Here's how the part is built. I have some questions about the finished solid (model axes, mm). Face numbers are marked on the shaded views. Coordinates: 2 decimals unless noted, no trailing zeros. Loops run counter-clockwise (first coordinate to the right, second up) from the corner with the lowest first, then second, coordinate; pieces in that order, holes last.
from build123d import *

# Parameters (mm, degrees)
F1_DEPTH  = 10.16
F2_W      = 208.28
F2_H      = 116.84
F3_DEPTH  = 0.254
F4_R      = 9.807477688
F4_R_2    = 8.537478745
F5_DEPTH  = 0.508
F6_DEPTH  = 0.254
F7_W      = 15.5448025422
F7_H      = 2.0574
F8_DEPTH  = 1.27
F9_DEPTH  = 0.254
F10_R     = 2.0193
F11_DEPTH = 0.762
F13_DEPTH = 2.54
F14_R     = 1.5445798635
F15_DEPTH = 2.54
F17_DEPTH = 76.2
F19_DEPTH = 0.762
F20_R     = 5.191457902
F20_R_2   = 3.4134577513
F21_DEPTH = 0.762
F22_DEPTH = 0.762
F23_R     = 2.6550671555
F24_DEPTH = 0.508


with BuildPart() as f1:
    # F0 (on Top) → F1 (new body)
    with BuildSketch(Plane.XY):
        with BuildLine():
            Line((-133.35, 0), (-133.35, -50.8))
            Line((-133.35, -50.8), (-133.35, -57.15))
            ThreePointArc((-133.35, -57.15), (-131.4901280605, -61.6401280605), (-127, -63.5))
            Line((-127, -63.5), (-120.65, -63.5))
            Line((-120.65, -63.5), (0, -63.5))
            Line((0, -63.5), (0, 0))
            Line((0, 0), (-133.35, 0))
        make_face()
        with BuildLine():
            Line((-133.35, 50.8), (-133.35, 0))
            Line((-133.35, 0), (0, 0))
            Line((0, 0), (0, 63.5))
            Line((0, 63.5), (-120.65, 63.5))
            Line((-120.65, 63.5), (-127, 63.5))
            ThreePointArc((-127, 63.5), (-131.4901280605, 61.6401280605), (-133.35, 57.15))
            Line((-133.35, 57.15), (-133.35, 50.8))
        make_face()
        with BuildLine():
            Line((0, 63.5), (0, 0))
            Line((0, 0), (0, -63.5))
            Line((0, -63.5), (120.65, -63.5))
            Line((120.65, -63.5), (127, -63.5))
            ThreePointArc((127, -63.5), (131.4901280605, -61.6401280605), (133.35, -57.15))
            Line((133.35, -57.15), (133.35, -50.8))
            Line((133.35, -50.8), (133.35, 50.8))
            Line((133.35, 50.8), (133.35, 57.15))
            ThreePointArc((133.35, 57.15), (131.4901280605, 61.6401280605), (127, 63.5))
            Line((127, 63.5), (120.65, 63.5))
            Line((120.65, 63.5), (0, 63.5))
        make_face()
    extrude(amount=F1_DEPTH)

    # F2 (on face) → F3 (cut)
    with BuildSketch(Plane.XY.offset(10.16)):
        with Locations((-3.81, 0)):
            Rectangle(F2_W, F2_H)
    extrude(amount=-F3_DEPTH, mode=Mode.SUBTRACT)

    # F4 (on face) → F5 (cut)
    with BuildSketch(Plane.XY.offset(10.16)):
        with Locations((117.7119389176, 0)):
            Circle(F4_R)
        with Locations((117.7119389176, 0)):
            Circle(F4_R_2, mode=Mode.SUBTRACT)
    extrude(amount=-F5_DEPTH, mode=Mode.SUBTRACT)

    # F6 (cut): a face of the model
    f6_faces = [f1.faces().sort_by_distance(p)[0] for p in [
        (117.7119389176, 0, 10.16),
    ]]
    extrude(f6_faces, amount=-F6_DEPTH, mode=Mode.SUBTRACT)

    # F7 (on face) → F8 (cut)
    with BuildSketch(Plane.XZ.offset(63.5)):
        with Locations((-107.9641506076, 5.8332554431)):
            Rectangle(F7_W, F7_H)
        with Locations((-107.9641506076, 3.7758554431)):
            Rectangle(F7_W, F7_H)
    extrude(amount=-F8_DEPTH, mode=Mode.SUBTRACT)

    # F7 (on face) → F9 (cut)
    with BuildSketch(Plane.XZ.offset(63.5)):
        with Locations((-107.9641506076, 5.8332554431)):
            Rectangle(F7_W, F7_H)
    extrude(amount=-F9_DEPTH, mode=Mode.SUBTRACT)

    # F10 (on face) → F11 (join)
    with BuildSketch(Plane.XZ.offset(63.5)):
        with Locations((-78.8557493365, 4.8045554431)):
            Circle(F10_R)
        with Locations((-89.5237493365, 4.8045554431)):
            Circle(F10_R)
    extrude(amount=F11_DEPTH)

    # F12 (on face) → F13 (cut)
    with BuildSketch(Plane.XY.offset(10.16)):
        Polygon((-120.4414889216, 17.2302983701), (-123.5122457147, 17.2302983701), (-123.5122457147, 0), (-123.5122457147, -17.2302983701), (-120.4414889216, -17.2302983701), (-120.4414889216, 0), align=None)
    extrude(amount=-F13_DEPTH, mode=Mode.SUBTRACT)

    # F14 (on face) → F15 (cut)
    with BuildSketch(Plane.XY.offset(10.16)):
        with Locations((-121.9860687852, -24.1657830775)):
            Circle(F14_R)
    extrude(amount=-F15_DEPTH, mode=Mode.SUBTRACT)

    # F16 (on face) → F17 (cut)
    with BuildSketch(Plane.YZ.offset(133.35)):
        Polygon((-9.0773701668, 3.7233135663), (0, 3.7233135663), (9.0773701668, 3.7233135663), (9.0773701668, 6.5667750314), (0, 6.5667750314), (-9.0773701668, 6.5667750314), align=None)
    extrude(amount=-F17_DEPTH, mode=Mode.SUBTRACT)

    # F18 (on face) → F19 (join)
    with BuildSketch(Plane(origin=(0, 63.5, 0), x_dir=(-1, 0, 0), z_dir=(0, 1, 0))):
        Polygon((98.232159481, 7.4123111553), (75.372159481, 7.4123111553), (75.372159481, 5.08), (75.372159481, 2.7476888447), (91.6486978531, 2.7476888447), (98.232159481, 2.7476888447), (98.232159481, 5.08), align=None)
    extrude(amount=F19_DEPTH)

    # F20 (on face) → F21 (join)
    with BuildSketch(Plane(origin=(0, 0, 0), x_dir=(1, 0, 0), z_dir=(0, 0, -1))):
        with Locations((-127, -55.3290322423)):
            Circle(F20_R)
        with Locations((-127, -55.3290322423)):
            Circle(F20_R_2, mode=Mode.SUBTRACT)
    extrude(amount=F21_DEPTH)

    # F20 (on face) → F22 (join)
    with BuildSketch(Plane(origin=(0, 0, 0), x_dir=(1, 0, 0), z_dir=(0, 0, -1))):
        with Locations((-127, -55.3290322423)):
            Circle(F20_R)
        with Locations((-127, -55.3290322423)):
            Circle(F20_R_2, mode=Mode.SUBTRACT)
    extrude(amount=F22_DEPTH)

    # F23 (on face) → F24 (join)
    with BuildSketch(Plane(origin=(0, 0, 0), x_dir=(1, 0, 0), z_dir=(0, 0, -1))):
        with Locations((-127.2339522839, -43.4491336346)):
            Circle(F23_R)
    extrude(amount=F24_DEPTH)


solid = f1.part
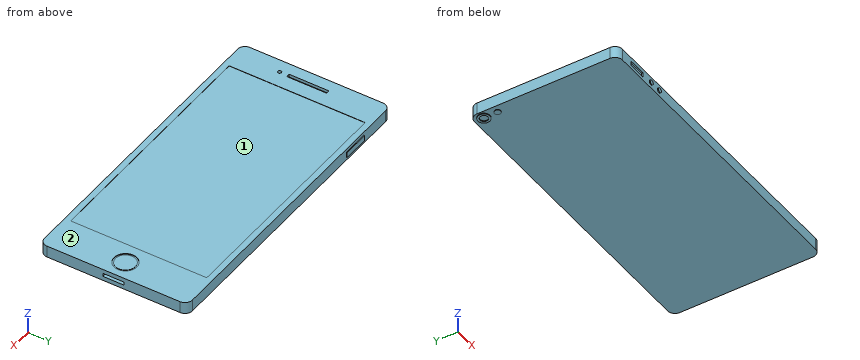
Q1. We'd pull the mould along Y, two halves only. Please class the marked faces 1 and 2: pulls with the +Y half, pulls with the -Y half, needs draft (parallel to the pull), parting line crosses it, or undercut.
Q2. Suppose I cut it at B-B on x = 20.5. Write out the boundary of the cut face in (y, z), and give its area (3 significant figures).
Q3. Suppose I cut it at D-D on y = -39. Write out the boundary of the cut face in (x, z).
Q4. Suppose I cut it at A-A on y = 0. Write out the boundary of the cut face in (x, z), and give its area (3 significant figures).
Q5. Suppose I cut it at C-C on y = 13. Write out the boundary of the cut face in (x, z), and give its area (3 significant figures).
Q6. Will these pins go through, and if not, where does the flat tip stop? P1, Ø1.5, axis at x = -19.5, y = 50.5, coming from the -Z side; P2, Ø3, axis at x = 59, z = 6, coming from the +Y side; P3, Ø1.5, axis at x = 85, z = 6, coming from the -Y side.
Q7. Please list where these lines run through material, in increasing order: probe 1 along Y at (x, z) = (-127, -0.4); probe 2 along X at (y, z) = (-16, 9.5); probe 3 along Y at (x, z) = (-111.5, 3.75).
Check values:
1. face 1: undercut
1. face 2: needs draft
2. outline: (-63.5, 0) - (63.5, 0) - (63.5, 10.16) - (58.42, 10.16) - (58.42, 9.91) - (-58.42, 9.91) - (-58.42, 10.16) - (-63.5, 10.16) - close
2. area: 1,260 mm2
3. outline: (-133.35, 0) - (133.35, 0) - (133.35, 10.16) - (100.33, 10.16) - (100.33, 9.91) - (-107.95, 9.91) - (-107.95, 10.16) - (-133.35, 10.16) - close
4. outline: (-133.35, 0) - (133.35, 0) - (133.35, 3.72) - (57.15, 3.72) - (57.15, 6.57) - (133.35, 6.57) - (133.35, 10.16) - (127.52, 10.16) - (127.52, 9.65) - (126.25, 9.65) - (126.25, 9.91) - (109.17, 9.91) - (109.17, 9.65) - (107.9, 9.65) - (107.9, 10.16) - (100.33, 10.16) - (100.33, 9.91) - (-107.95, 9.91) - (-107.95, 10.16) - (-120.44, 10.16) - (-120.44, 7.62) - (-123.51, 7.62) - (-123.51, 10.16) - (-133.35, 10.16) - close
4. area: 2,430 mm2
5. outline: (-133.35, 0) - (133.35, 0) - (133.35, 10.16) - (100.33, 10.16) - (100.33, 9.91) - (-107.95, 9.91) - (-107.95, 10.16) - (-120.44, 10.16) - (-120.44, 7.62) - (-123.51, 7.62) - (-123.51, 10.16) - (-133.35, 10.16) - close
5. area: 2,650 mm2
6. P1: stops at z = 0
6. P2: stops at y = 63.5
6. P3: stops at y = -63.5
7. probe 1: y = 40.8 to 46.09, 50.14 to 51.92, 58.74 to 60.52
7. probe 2: x = -133.35 to -123.51, -120.44 to 133.35
7. probe 3: y = -62.23 to 63.5
